Could you check a few things on this model? Use its own coordinates, in mm. Face numbers are marked on the shaded views. A direction names the side the tool comes from. Give positions to 0.01 mm unless a question says otherwise; leave off trailing zeros. Order: outer loops, then holes, each group sorted by start corner. A loop starts at its lowest first (then second) coordinate and runs counter-clockwise, first axis right, second up. Notation, with made-up numbers: M -36.75,74.25 L 2.25,74.25 A22 cw 2.25,110.25 Z; hole C -17.5,-4.75 d2. An arc over 180 degrees is marked long. Answer in a Markdown table with one row per item. Add a question column.
```python
from build123d import *

# Parameters (mm, degrees)
BOSS_EXTRUDE1_DEPTH = 44.45
SKETCH2_R           = 5.499261314
SKETCH2_R_2         = 4.7625
CUT_EXTRUDE1_DEPTH  = 7.9375
SKETCH3_R           = 5.499261314
SKETCH3_R_2         = 4.7625
CUT_EXTRUDE2_DEPTH  = 7.9375


with BuildPart() as part:
    # Sketch1 → Boss-Extrude1 (new body)
    with BuildSketch(Plane(origin=(0, 0, 0), x_dir=(0, 0, -1), z_dir=(1, 0, 0))):
        Polygon((0, 5.499261314), (-4.7625, 2.749630657), (-4.7625, -2.749630657), (0, -5.499261314), (4.7625, -2.749630657), (4.7625, 2.749630657), align=None)
    extrude(amount=BOSS_EXTRUDE1_DEPTH)

    # Sketch2 → Cut-Extrude1 (cut)
    with BuildSketch(Plane.ZY):
        Circle(SKETCH2_R)
        Circle(SKETCH2_R_2, mode=Mode.SUBTRACT)
    extrude(amount=-CUT_EXTRUDE1_DEPTH, mode=Mode.SUBTRACT)

    # Sketch3 → Cut-Extrude2 (cut)
    with BuildSketch(Plane(origin=(44.45, 0, 0), x_dir=(0, 0, -1), z_dir=(1, 0, 0))):
        Circle(SKETCH3_R)
        Circle(SKETCH3_R_2, mode=Mode.SUBTRACT)
    extrude(amount=-CUT_EXTRUDE2_DEPTH, mode=Mode.SUBTRACT)


solid = part.part
```
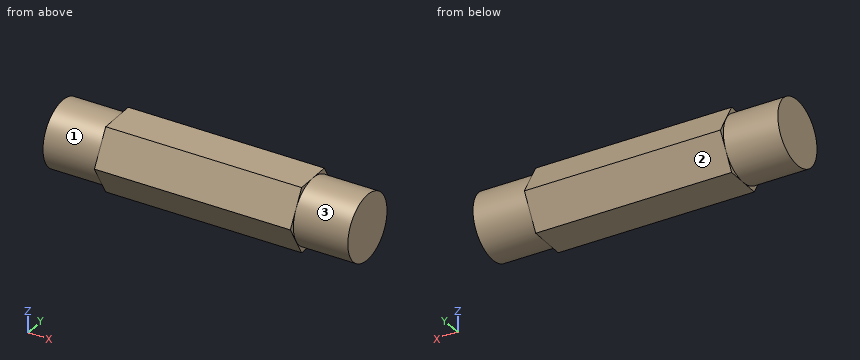
1. Suppose I cut it at A-A on z = 3.25. List the corners of the cut face in (x, y) for me.
2. Suppose I cut it at D-D on x = 37.5. List the corners of the cut face in (y, z) for me (1 decimal).
3. For the marked faces 1, 2 and 3, which set-ups out of +Z, -Z, +X, -X, +Y, -Y let a thin tool reach every point of the face, with its end or its side?
4. Suppose I cut it at B-B on y = 2. List the corners of the cut face in (x, z) for me, plus the area to 3 significant figures.
5. If I drill on line 1 along Y through (x, z) = (13.5, 0.5); line 2 along Y through (x, z) = (40.5, 2.75); line 3 along Z through (x, y) = (27, 4), over which ranges is the centre line in solid material (lowest first)? Write a range as [from, to].
6. Suppose I cut it at C-C on x = 33. List the corners of the cut face in (y, z) for me, plus the area to 3 significant figures.
7. Will this pin go through, and if not, where does the flat tip stop? P1, Ø5, axis at x = 24, z = -1, coming from the -Y side.
Findings below:
| question | item | result |
|---|---|---|
| 1 | outline | M 0,-3.48 L 7.94,-3.48 L 7.94,-3.62 L 36.51,-3.62 L 36.51,-3.48 L 44.45,-3.48 L 44.45,3.48 L 36.51,3.48 L 36.51,3.62 L 7.94,3.62 L 7.94,3.48 L 0,3.48 Z |
| 2 | outline | C 0,0 d9.5 |
| 3 | face 1 | -X |
| 3 | face 2 | -Z, +X, -X, +Y |
| 3 | face 3 | +X |
| 4 | outline | M 0,-4.32 L 7.94,-4.32 L 7.94,-4.76 L 36.51,-4.76 L 36.51,-4.32 L 44.45,-4.32 L 44.45,4.32 L 36.51,4.32 L 36.51,4.76 L 7.94,4.76 L 7.94,4.32 L 0,4.32 Z |
| 4 | area | 409 mm2 |
| 5 | line 1 | [-5.21, 5.21] |
| 5 | line 2 | [-3.89, 3.89] |
| 5 | line 3 | [-2.6, 2.6] |
| 6 | outline | M -5.5,0 L -2.75,-4.76 L 2.75,-4.76 L 5.5,0 L 2.75,4.76 L -2.75,4.76 Z |
| 6 | area | 78.6 mm2 |
| 7 | P1 | y = -5.5 |
